Autodesk Inventor part; units mm, degrees
ref_plane "Work Plane1" through (1.525, 0, 0) normal (0, 0, 1) x (1, 0, 0)
ref_plane "YZ Plane" through (0, 0, 0) normal (1, 0, 0) x (0, 1, 0)
ref_plane "XZ Plane" through (0, 0, 0) normal (0, 1, 0) x (-1, 0, 0)
sketch "Sketch1" plane through (0, 0, 0) normal (0, 0, 1) x (1, 0, 0)
  line L0 (0, 5) -> (0, 3)
  line L1 (3, 3) -> (12, 3)
  line L2 (12, 3) -> (12, 0)
  line L3 (12, 0) -> (-0.5001, 0)
  line L4 (-3.0001, 0) -> (14.5, 0)
  line L5 (-0.5001, 0) -> (-0.5001, 5)
  line L6 (-0.5001, 5) -> (0, 5)
  line L7 (3, 3) -> (2.3865, 3)
  line L8 (2.3865, 3) -> (0, 3)
  line L9 (0, -1) -> (0, 6)
  dimension "d0" = 12
  dimension "d1" = 9
  dimension "d2" = 6
  dimension "d9" = 0.5001
  dimension "d10" = 10
  dimension "d13" = 0.6136
  dimension "d14" = 6
revolve "Body" add sketch "Sketch1" angle 360 about axis through (12, 0, 0) along (-1, 0, 0)
sketch "Sketch2" plane through (-0.5001, 0, 0) normal (-1, 0, 0) x (0, 0, 1)
  line L0 (0, 5.7735) -> (5, 2.8868)
  line L1 (5, 2.8868) -> (5, -2.8868)
  line L2 (5, -2.8868) -> (0, -5.7735)
  line L3 (0, -5.7735) -> (-5, -2.8868)
  line L4 (-5, -2.8868) -> (-5, 2.8868)
  line L5 (-5, 2.8868) -> (0, 5.7735)
  point P0 (0, 0)
  point P1 (0, 0)
  dimension "d11" = 10
extrude "Head" add sketch "Sketch2" along normal blind 3.5
sketch "Sketch4" plane through (0, 0, 0) normal (0, 0, 1) x (1, 0, 0)
  line L0 (-4.0001, 5) -> (-4.0001, 5.7735)
  line L1 (-4.0001, 5.7735) -> (-3.5535, 5.7735)
  line L2 (-3.5535, 5.7735) -> (-4.0001, 5)
  line L3 (-4.7001, 0) -> (0.1999, 0)
  line L4 (-0.5001, 5.7735) -> (-4.0001, 5.7735)
  line L5 (-4.0001, 2.8868) -> (-4.0001, 5.7735)
  dimension "d5" = 30
  dimension "d19" = 10
revolve "Chamfer1" cut sketch "Sketch4" angle 360 about axis through (-10, 0, 0) along (1, 0, 0)
thread "Thread"
chamfer "Chamfer2" distance 0.6135 distance2 0.6136 1 edges at (12, -3, 0) measured on face at (12, -0.5681, 0.823)
ref_plane "Work Plane1" through (1.525, 0, 0) normal (0, 0, 1) x (1, 0, 0)
equation "\"d11\" = SW"
equation "\"d3\" = KOH - SD"
equation "\"d15\" = GEL"
equation "\"d6\" = -0.5 * SPD + 0.5 * GD"
equation "\"d0\" = NLG"
equation "\"d1\" = GEL"
equation "\"d2\" = GD"
equation "\"d10\" = SD2"
equation "\"d14\" = BDM"
equation "\"d5\" = ANG1"
equation "\"d19\" = SW0"
equation "\"NLG\" = 12"
equation "\"GD\" = NND"
equation "\"BDM\" = NND"
equation "\"KOH\" = 4"
equation "\"GEL\" = 9"
equation "\"SW\" = 10"
equation "\"SW0\" = SW"
equation "\"SPD\" = NND - 1.2269 * PTC"
equation "\"SD2\" = SW"
equation "\"SD\" = 0.5"
equation "\"ANG1\" = 30deg"
equation "\"GAL\" = 0.61345 * PTC"
equation "\"GUL\" = 0.61345 * PTC"
equation "\"RR\" = 0.25"
equation "\"WFT\" = SD"
equation "\"GD1\" = THREADDIA - 1.2269 * PTC"
equation "\"THREADDIA\" = 6"
equation "\"TOA\" = 30deg"
equation "\"FAWI\" = 45deg"
equation "\"PTC\" = 1"
equation "\"NND\" = 6"
equation "\"E0\" = 1.155 * SW"
properties part number "AS 1110 - M6 x 12" material "Steel, Mild"
Here's how the part is built. I have some questions about the finished solid (model axes, mm). A direction names the side the tool comes from. Coordinates: 2 decimals unless noted, no trailing zeros. Loops run counter-clockwise (first coordinate to the right, second up) from the corner with the lowest first, then second, coordinate; pieces in that order, holes last.
1. I need wall thicknesses on L1, parallel to X at y = 3.5, z = 3.25; L2, parallel to Z at x = 1.25, y = 2; L3, parallel to Y at x = 8.5, z = -2.75. Which ranges of each line are inside material? Lowest first, please.
2. For P1, Ø1.3, axis at y = -3, z = 4, coming from the +X side; P2, Ø4, axis at x = 7.5, z = -3, coming from the -Y side; P3, Ø1.5, axis at x = 3.5, y = 3.5, coming from the -Z side, each with a flat end and sliding along its axis, tell me the tip position at first contact or that it passes through.
3. For faces 1 (the flat face through (-0.5, -5.2, 0)), 2 (the flat face through (-0.5, -2.6, 4.5)), 3 (the flat face through (-0.5, 2.7, -4.5)), 4 (the cylindrical face through (6, -3, 0)), 5 (the flat face through (-0.5, 2.7, 4.5)), which set-ups out of +Z, -Z, +X, -X, +Y, -Y let a thin tool reach every point of the face, with its end or its side?
4. Imagine slicing it at A-A, the plane x = 10.5. Please give me the cut outline in (y, z), and give its area (3 significant figures).
Taken from the geometry:
1. L1: x = -4 to 0
1. L2: z = -2.24 to 2.24
1. L3: y = -1.2 to 1.2
2. P1: stops at x = 0
2. P2: stops at y = -2.83
2. P3: stops at z = -1.2
3. face 1: +X, -Y
3. face 2: +Z, +X, -Y
3. face 3: -Z, +X, +Y
3. face 4: +X
3. face 5: +Z, +X, +Y
4. outline: circle Ø6 at (0, 0)
4. area: 28.3 mm2
